Can you work these out from the drawing? Everything is in mm from the part's minimum corner. Give positions to 0.01 mm unless a question says otherwise; leave off trailing zeros. Write each loop counter-clockwise with the first axis right and the second up, starting at its lowest first coordinate (ties: lowest second). Pieces come first, ordered by that corner, then holes. Notation, with made-up numbers: (71.25, 0) - (95.25, 0) arc R25 ccw to (95.25, 33) - close; hole circle Ø5 at (40.25, -19.5). An arc over 180 degrees is marked (long way). Use a Markdown table: item, result.
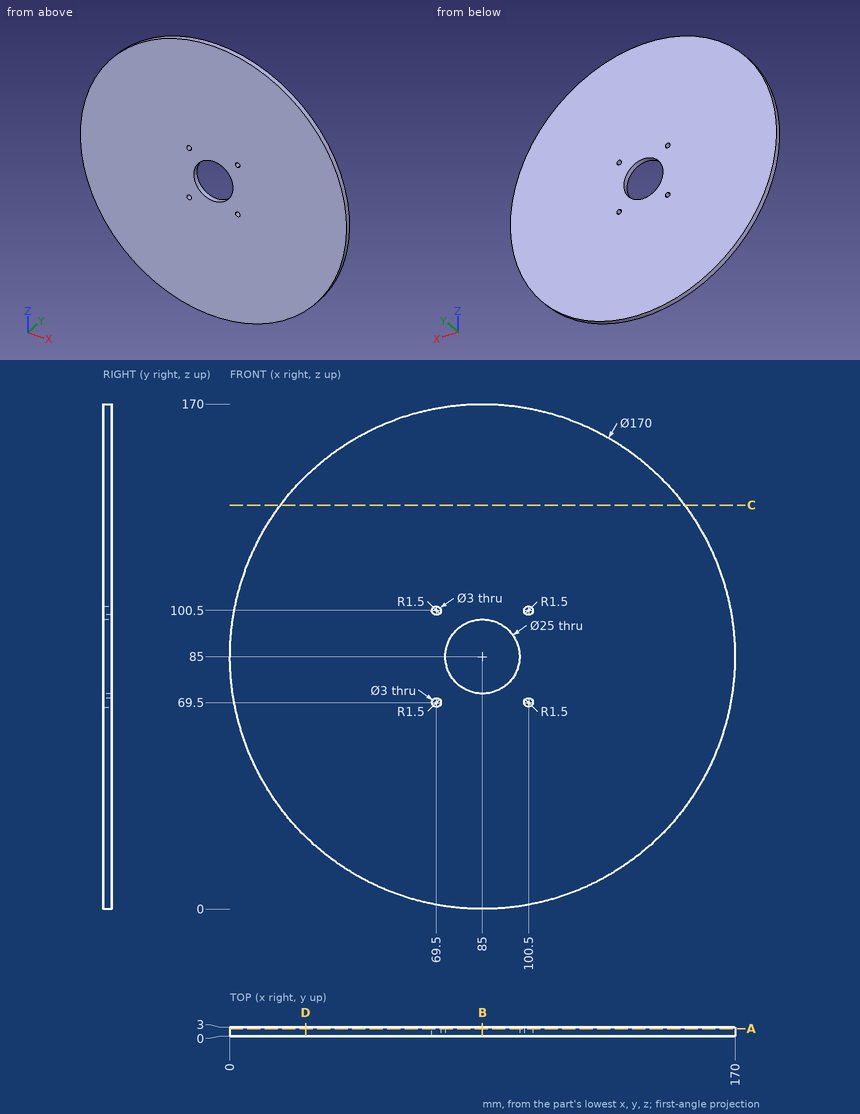
Item 1: Will this pin go through, and if not, where does the flat tip stop? pin 1 Ø3.5 at (x, z) = (69.5, 100.5) entering from -Y.
Values:
| item | result |
|---|---|
| pin 1 | stops at y = 0 |
Item 2: If we section it at B-B, the plane x = 85: Write out the boundary of the cut face in (y, z), plus the area to 3 significant figures.
Values:
| item | result |
|---|---|
| outline | (0, 0) - (3, 0) - (3, 72.5) - (0, 72.5) - close; (0, 97.5) - (3, 97.5) - (3, 170) - (0, 170) - close |
| area | 435 mm2 |
Item 3: If we section it at A-A, the plane y = 2.45: Write out the boundary of the cut face in (x, z), plus the area to 3 significant figures.
Values:
| item | result |
|---|---|
| outline | circle Ø170 at (85, 85); hole circle Ø3 at (69.5, 69.5); hole circle Ø3 at (69.5, 100.5); hole circle Ø25 at (85, 85); hole circle Ø3 at (100.5, 69.5); hole circle Ø3 at (100.5, 100.5) |
| area | 22,200 mm2 |
Item 4: If we section it at C-C, the plane z = 136: Write out the boundary of the cut face in (x, y), plus the area to 3 significant figures.
Values:
| item | result |
|---|---|
| outline | (17, 0) - (153, 0) - (153, 3) - (17, 3) - close |
| area | 408 mm2 |
Item 5: I need wall thicknesses on line 1 along Z through (x, y) = (85.5, 1.4); line 2 along Z through (x, y) = (101.5, 0.5); line 3 along X through (y, z) = (1, 69.5). Which ranges of each line are inside material? Lowest first, please. Write a range as [from, to].
Values:
| item | result |
|---|---|
| line 1 | z = [0, 72.51], [97.49, 170] |
| line 2 | z = [1.62, 68.38], [70.62, 99.38], [101.62, 168.38] |
| line 3 | x = [1.43, 68], [71, 99], [102, 168.57] |
Item 6: If we section it at D-D, the plane x = 25.5: Write out the boundary of the cut face in (y, z).
Values:
| item | result |
|---|---|
| outline | (0, 24.3) - (3, 24.3) - (3, 145.7) - (0, 145.7) - close |
